from build123d import *

# Parameters (mm, degrees)
F_1_2_13_TAPPED_HOLE1_D     = 10.71626
F_1_2_13_TAPPED_HOLE1_DEPTH = 19.05
F_1_2_13_TAPPED_HOLE1_TIP   = 3.219489309


with BuildPart() as part:
    # Sketch1 → Revolve1 (revolve)
    with BuildSketch(Plane.XY):
        with BuildLine():
            Line((0, 0), (0, 43.6753))
            Line((0, 43.6753), (8.73125, 43.6753))
            ThreePointArc((8.73125, 43.6753), (9.292516008, 43.442816008), (9.525, 42.88155))
            Line((9.525, 42.88155), (9.525, 0.79375))
            Line((9.525, 0.79375), (9.525, 0))
            Line((9.525, 0), (0, 0))
        make_face()
    revolve(axis=Axis((0, 288.392157732, 0), (0, -1, 0)))

    # 1/2-13 Tapped Hole1
    with Locations(Plane(origin=(0, 43.6753, 0), x_dir=(1, 0, 0), z_dir=(0, 1, 0))):
        with Locations((0, 0)):
            Hole(F_1_2_13_TAPPED_HOLE1_D / 2, depth=F_1_2_13_TAPPED_HOLE1_DEPTH)
            with Locations((0, 0, -(F_1_2_13_TAPPED_HOLE1_DEPTH + F_1_2_13_TAPPED_HOLE1_TIP / 2))):  # 118° drill point
                Cone(0, F_1_2_13_TAPPED_HOLE1_D / 2, F_1_2_13_TAPPED_HOLE1_TIP, mode=Mode.SUBTRACT)

    # Mirror1: part across plane


with BuildPart() as part_1:
    add(part.part)
    add(part.part.mirror(Plane.ZX))


solid = part_1.part
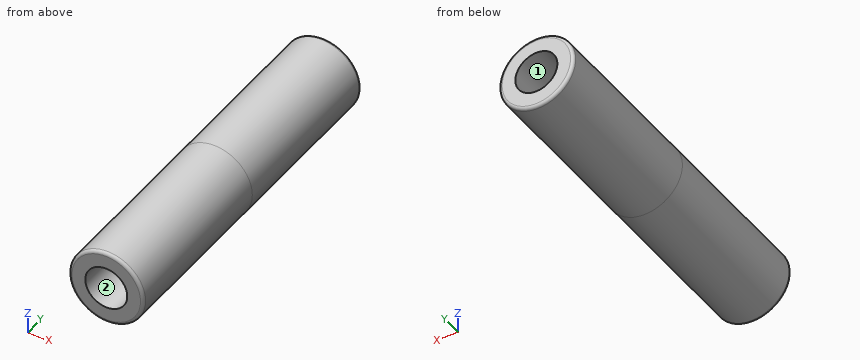
CAD build for the part. Positions are in the model's coordinates, mm. Face numbers are marked on the shaded views. Give positions to 0.01 mm unless a question says otherwise; leave off trailing zeros. Loops run counter-clockwise (first coordinate to the right, second up) from the corner with the lowest first, then second, coordinate; pieces in that order, holes last. Notation, with made-up numbers: M -11,29 L -3,29 A13 cw -3,36 Z; hole C 59,-16 d1. An arc over 180 degrees is marked long. Answer in a Markdown table with one row per item. Add a question column.
Item 1: Mould opens along Z. For the marked faces 1 and 2 say: +Z half, -Z half, draft (parallel to the pull), parting line (faces both ways), or undercut.
Item 2: Probe probe 1 along Z at (x, y) = (0, 34.5) (3 decimals); probe 2 along Z at (x, y) = (3.5, -30); probe 3 along X at (y, z) = (29, 2.75). List the from-to ranges inside material, lowest first.
Item 3: Drop flat-ended pins along their axis: P1, Ø3, axis at x = 0, z = -4.5, coming from the -Y side; P2, Ø8, axis at x = -5.5, y = -13, coming from the +Z side; P3, Ø4, axis at y = -8, z = -6.5, coming from the +X side (3 decimals); P4, Ø6, axis at x = 4, y = -1, coming from the +Z side. Give the stop position or say it passes through.
Item 4: Band-saw the part on A-A on y = -30.5. Give the cut face in (x, z) (3 decimals).
Item 5: Band-saw the part on B-B on y = 2. Give the cut face in (x, z) (3 decimals), then the cut area to 3 significant figures.
Reply:
| question | item | result |
|---|---|---|
| 1 | face 1 | undercut |
| 1 | face 2 | undercut |
| 2 | probe 1 | z = -9.525 to -5.358, 5.358 to 9.525 |
| 2 | probe 2 | z = -8.86 to -4.06, 4.06 to 8.86 |
| 2 | probe 3 | x = -9.12 to -4.6, 4.6 to 9.12 |
| 3 | P1 | stops at y = -43.68 |
| 3 | P2 | stops at z = 9.41 |
| 3 | P3 | stops at x = 8.395 |
| 3 | P4 | stops at z = 9.47 |
| 4 | outline | C 0,0 d19.05; hole C 0,0 d10.716 |
| 5 | outline | C 0,0 d19.05 |
| 5 | area | 285 mm^2 |
